Autodesk Inventor part; units mm, degrees
ref_plane "YZ Plane" through (0, 0, 0) normal (1, 0, 0) x (0, 1, 0)
ref_plane "XZ Plane" through (0, 0, 0) normal (0, 1, 0) x (-1, 0, 0)
ref_plane "XY Plane" through (0, 0, 0) normal (0, 0, 1) x (1, 0, 0)
sketch "Sketch1" plane through (0, 0, 0) normal (0, 1, 0) x (-1, 0, 0)
  line L0 (0, 0) -> (914.4, 0)
  line L1 (914.4, 0) -> (914.4, -609.6)
  line L2 (914.4, -609.6) -> (0, -609.6)
  line L3 (0, -609.6) -> (0, 0)
  line L4 (0, -609.6) -> (76.2, -609.6)
  line L5 (76.2, -609.6) -> (76.2, -533.4)
  line L6 (76.2, -533.4) -> (0, -533.4)
  line L7 (0, -533.4) -> (0, -609.6)
  line L8 (0, 0) -> (76.2, 0)
  line L9 (76.2, 0) -> (76.2, -76.2)
  line L10 (76.2, -76.2) -> (0, -76.2)
  line L11 (0, -76.2) -> (0, 0)
  line L12 (914.4, -609.6) -> (838.2, -609.6)
  line L13 (838.2, -609.6) -> (838.2, -533.4)
  line L14 (838.2, -533.4) -> (914.4, -533.4)
  line L15 (914.4, -533.4) -> (914.4, -609.6)
  line L16 (914.4, 0) -> (838.2, 0)
  line L17 (838.2, 0) -> (838.2, -76.2)
  line L18 (838.2, -76.2) -> (914.4, -76.2)
  line L19 (914.4, -76.2) -> (914.4, 0)
  arc A0 (838.2, -571.5) -> (76.2, -571.5) centre (457.2, -1079.5) ccw
  arc A1 (76.2, -38.1) -> (838.2, -38.1) centre (457.2, 469.9) ccw
  arc A2 (876.3, -76.2) -> (876.3, -533.4) centre (1468.7247, -304.8) ccw
  arc A3 (38.1, -533.4) -> (38.1, -76.2) centre (-554.3247, -304.8) ccw
  dimension "d17" = 609.6
  dimension "d18" = 76.2
  dimension "d19" = 76.2
  dimension "d20" = 76.2
  dimension "d21" = 76.2
  dimension "d22" = 76.2
  dimension "d23" = 76.2
  dimension "d24" = 76.2
  dimension "d25" = 76.2
  dimension "d26" = 635
  dimension "d27" = 635
  dimension "d28" = 635
  dimension "d29" = 635
extrude "Extrusion2" add sketch "Sketch1" along normal blind 6.35 contours L0 L9 L10 L3 | L0 L1 L18 L17 | A1 L17 L18 A2 L14 L13 A0 L5 L6 A3 L10 L9 | L6 L5 L2 L3 | L1 L2 L13 L14
sketch "Sketch2" plane through (0, 6.35, 0) normal (0, 1, 0) x (1, 0, 0)
  arc A0 (-76.2, 38.1) -> (-838.2, 38.1) centre (-457.2, -469.9) ccw
  arc A1 (-838.2, 571.5) -> (-76.2, 571.5) centre (-457.2, 1079.5) ccw
  line L0 (-457.2, 304.8) -> (-457.2, 241.3)
  line L1 (-457.2, 241.3) -> (-584.2, 241.3)
  line L2 (-584.2, 241.3) -> (-584.2, 368.3)
  line L3 (-584.2, 368.3) -> (-457.2, 368.3)
  line L4 (-457.2, 368.3) -> (-457.2, 241.3)
  line L5 (-584.2, 304.8) -> (-520.7, 368.3) construction
  line L6 (-520.7, 368.3) -> (-457.2, 304.8) construction
  line L7 (-552.45, 336.55) -> (-488.95, 336.55) construction
  line L8 (-584.2, 304.8) -> (-520.7, 241.3) construction
  line L9 (-457.2, 304.8) -> (-520.7, 241.3) construction
  line L10 (-552.45, 273.05) -> (-488.95, 273.05) construction
  circle A2 centre (-552.45, 273.05) radius 4.5 construction
  circle A3 centre (-488.95, 273.05) radius 4.5 construction
  circle A4 centre (-488.95, 336.55) radius 4.5 construction
  circle A5 centre (-552.45, 336.55) radius 4.5 construction
  point P0 (0, 0)
  dimension "d35" = 9
  dimension "d36" = 9
  dimension "d37" = 9
  dimension "d38" = 9
hole "Hole1" at (-552.45, 6.35, -273.05) at (-552.45, 6.35, -336.55) at (-488.95, 6.35, -336.55) at (-488.95, 6.35, -273.05) direction (0, -1, 0) diameter 10.5918 end through all
sketch "Sketch3" plane through (0, 6.35, 0) normal (0, 1, 0) x (1, 0, 0)
  point P0 (0, 0)
sketch "Sketch4" plane through (0, 6.35, 0) normal (0, 1, 0) x (1, 0, 0)
  line L0 (-401.2293, 193.7971) -> (-99.5943, 193.7971)
  line L1 (-99.5943, 193.7971) -> (-99.5943, 428.1144)
  line L2 (-99.5943, 428.1144) -> (-401.2293, 428.1144)
  line L3 (-401.2293, 428.1144) -> (-401.2293, 193.7971)
  point P0 (0, 0)
extrude "Extrusion3" cut sketch "Sketch4" against normal blind 6.35
properties part number "TopV3"
Work out the finished part from the listing and answer in its coordinate system (mm). Coordinates: 2 decimals unless noted, no trailing zeros. Order: outer loops, then holes, each group sorted by start corner. A loop starts at its lowest first (then second) coordinate and runs counter-clockwise, first axis right, second up. Notation, with made-up numbers: (-35, 2) - (-17, 2) arc R25 cw to (-17, 17) - close; hole circle Ø6 at (18, -16). An arc over 180 degrees is marked (long way). Put each result on its own line as item: value. Start each with the question number.
1) Find section B-B (y = 3.5). Give the vertices of the cut face in (x, z), plus the area to 3 significant figures.
2) Find section D-D (x = -572). Give the vertices of the cut face in (y, z), plus the area to 3 significant figures.
3) Find the intervals of material crossed by line 1 (X direction, y = 5, z = -333); line 2 (X direction, y = 5, z = -336.55); line 3 (Z direction, x = -488.95, y = 3.75), in increasing order. Write a range as from..to.
4) Find section C-C (x = -188). Give the vertices of the cut face in (y, z), plus the area to 3 significant figures.
5) Find section A-A (z = -353). Give the vertices of the cut face in (x, y), plus the area to 3 significant figures.
6) Flat-ended cylindrical pins translate along their axes: pin 1 (3 mm diameter, centred on y = 2, z = -423, fed in from -X); pin 2 (1.9 mm diameter, centred on x = -250.5, y = 2, fed in from +Z). Find the tip coordinate at first contact, or state that the pin passes through.
7) For a pull along X with two mould halves and no side action, classify faces 1 (the flat face through (-552, 6.35, -301)), 2 (the cylindrical face through (-80.667, 3.131, -301.526)), 3 (the cylindrical face through (-451.479, 3.131, -444.526)), 4 (the cylindrical face through (-833.733, 3.131, -308.074)) as released by +X, released by -X, zero draft, split by the parting line, or undercut.
Results list:
1. outline: (-914.4, -609.6) - (-838.2, -609.6) - (-838.2, -571.5) arc R635 cw to (-76.2, -571.5) - (-76.2, -609.6) - (0, -609.6) - (0, -533.4) - (-38.1, -533.4) arc R635 cw to (-38.1, -76.2) - (0, -76.2) - (0, 0) - (-76.2, 0) - (-76.2, -38.1) arc R635 cw to (-838.2, -38.1) - (-838.2, 0) - (-914.4, 0) - (-914.4, -76.2) - (-876.3, -76.2) arc R635 cw to (-876.3, -533.4) - (-914.4, -533.4) - close; hole circle Ø10.59 at (-552.45, -336.55); hole circle Ø10.59 at (-552.45, -273.05); hole circle Ø10.59 at (-488.95, -336.55); hole circle Ø10.59 at (-488.95, -273.05); hole (-401.23, -428.11) - (-99.59, -428.11) - (-99.59, -193.8) - (-401.23, -193.8) - close
1. area: 235,000 mm^2
2. outline: (0, -454.96) - (6.35, -454.96) - (6.35, -154.64) - (0, -154.64) - close
2. area: 1,910 mm^2
3. line 1: x = -834.35..-556.38, -548.52..-492.88, -485.02..-401.23, -99.59..-80.05
3. line 2: x = -834.52..-557.75, -547.15..-494.25, -483.65..-401.23, -99.59..-79.88
3. line 3: z = -445.29..-341.85, -331.25..-278.35, -267.75..-164.31
4. outline: (0, -504.39) - (6.35, -504.39) - (6.35, -428.11) - (0, -428.11) - close; (0, -193.8) - (6.35, -193.8) - (6.35, -105.21) - (0, -105.21) - close
4. area: 1,050 mm^2
5. outline: (-835.56, 0) - (-401.23, 0) - (-401.23, 6.35) - (-835.56, 6.35) - close; (-99.59, 0) - (-78.84, 0) - (-78.84, 6.35) - (-99.59, 6.35) - close
5. area: 2,890 mm^2
6. pin 1: stops at x = -845.11
6. pin 2: stops at z = -130.19
7. face 1: zero draft
7. face 2: released by +X
7. face 3: undercut
7. face 4: released by -X
